The model under review builds one solid part; all positions refer to its coordinate system, in mm. Face numbers are marked on the shaded views. A direction names the side the tool comes from. Coordinates: 2 decimals unless noted, no trailing zeros. Write each loop counter-clockwise with the first axis right and the second up, starting at its lowest first coordinate (ties: lowest second). Pieces come first, ordered by that corner, then holes.
1) Add section C-C, the plane x = 25. State the section outline as (y, z) points.
2) Add section A-A, the plane y = -12.5. State the section outline as (x, z) points.
3) For P1, Ø10, axis at x = 25.5, z = 15, coming from the -Y side (3 decimals); P2, Ø1.2, axis at y = 1, z = 23.5, coming from the +X side; P3, Ø2, axis at y = 0.5, z = 25, coming from the -X side; P4, Ø8, axis at x = 18.5, y = -19, coming from the +Z side, all flat-tipped, find the tip position at first contact; note any pin that passes through.
4) Add section D-D, the plane z = 20. State the section outline as (x, y) points.
5) Mouldability with a two-part tool opening along Z and no side actions: class the marked faces 4, 5 and 6 as released by +Z, released by -Z, zero draft, split by the parting line, or undercut.
6) For line 1 (X direction, y = 12.5, z = 1.5); line 2 (Y direction, x = -25, z = 4); line 3 (Y direction, x = 0, z = 39.6), list the stretches that pass through material, from the lowest coordinate up.
7) Add section B-B, the plane z = 3. State the section outline as (x, y) points, then the cut area to 3 significant figures.
8) Machinability: for the marked faces 1, 2 and 3, which of the approach directions +Z, -Z, +X, -X, +Y, -Y give a long, thin tool a straight path to every point of the face, cutting with its end or side? Answer none if there is none.
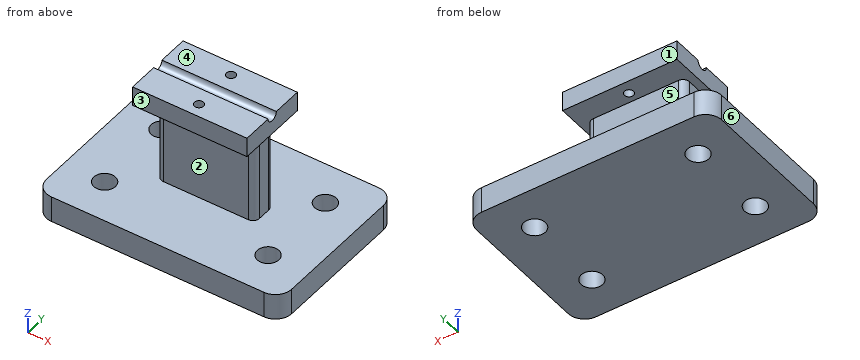
Autodesk Fusion 360 part; units mm, degrees
sketch "草图1" plane through (0, 0, 0) normal (0, 0, 1) x (1, 0, 0)
  line L0 (37.5, -25) -> (-37.5, -25)
  line L1 (-37.5, -25) -> (-37.5, 25)
  line L2 (-37.5, 25) -> (37.5, 25)
  line L3 (37.5, 25) -> (37.5, -25)
  line L4 (37.5, -25) -> (-37.5, 25) construction
  line L5 (-37.5, -25) -> (37.5, 25) construction
  dimension "d34" = 75
  dimension "d35" = 50
extrude "拉伸1" add sketch "草图1" along normal blind 8
fillet "圆角1" radius 5 4 edges at (37.5, -25, 4) (-37.5, -25, 4) (37.5, 25, 4) (-37.5, 25, 4)
sketch "草图2" plane through (0, 0, 8) normal (0, 0, 1) x (-1, 0, 0)
  arc A0 (32.5, -25) -> (37.5, -20) centre (32.5, -20) ccw
  line L0 (37.5, -20) -> (37.5, 20)
  arc A1 (37.5, 20) -> (32.5, 25) centre (32.5, 20) ccw
  line L1 (32.5, 25) -> (-32.5, 25)
  arc A2 (-32.5, 25) -> (-37.5, 20) centre (-32.5, 20) ccw
  line L2 (-37.5, 20) -> (-37.5, -20)
  arc A3 (-37.5, -20) -> (-32.5, -25) centre (-32.5, -20) ccw
  line L3 (-32.5, -25) -> (32.5, -25)
  point P0 (-25, -12.5)
  dimension "d40" = 12.5
  dimension "d41" = 12.5
hole "孔1" at (25, 12.5, 8) direction (0, 0, -1) diameter 6.6 depth 25 tip angle 180
pattern_linear "R-阵列1" count 2 spacing 50 along (-1, 0, 0) count 2 spacing 25 along (0, -1, 0) of "孔1"
sketch "草图3" plane through (0, 0, 8) normal (0, 0, 1) x (-1, 0, 0)
  circle A0 centre (25, 12.5) radius 3.3
  circle A1 centre (-25, 12.5) radius 3.3
  circle A2 centre (25, -12.5) radius 3.3
  circle A3 centre (-25, -12.5) radius 3.3
  arc A4 (32.5, -25) -> (37.5, -20) centre (32.5, -20) ccw
  line L0 (37.5, -20) -> (37.5, 20)
  arc A5 (37.5, 20) -> (32.5, 25) centre (32.5, 20) ccw
  line L1 (32.5, 25) -> (-32.5, 25)
  arc A6 (-32.5, 25) -> (-37.5, 20) centre (-32.5, 20) ccw
  line L2 (-37.5, 20) -> (-37.5, -20)
  arc A7 (-37.5, -20) -> (-32.5, -25) centre (-32.5, -20) ccw
  line L3 (-32.5, -25) -> (32.5, -25)
  line L4 (15, -4) -> (-15, -4)
  line L5 (-15, -4) -> (-15, 4)
  line L6 (-15, 4) -> (15, 4)
  line L7 (15, 4) -> (15, -4)
  line L8 (15, -4) -> (-15, 4) construction
  line L9 (-15, -4) -> (15, 4) construction
  dimension "d49" = 30
  dimension "d50" = 8
extrude "拉伸2" add sketch "草图3" along normal blind 27.5 contours L4 L5 L6 L7
sketch "草图4" plane through (0, 0, 35.5) normal (0, 0, 1) x (-1, 0, 0)
  line L0 (15, 4) -> (-15, 4)
  line L1 (-15, 4) -> (-15, -4)
  line L2 (-15, -4) -> (15, -4)
  line L3 (15, -4) -> (15, 4)
  line L4 (17.5, -11) -> (-17.5, -11)
  line L5 (-17.5, -11) -> (-17.5, 11)
  line L6 (-17.5, 11) -> (17.5, 11)
  line L7 (17.5, 11) -> (17.5, -11)
  line L8 (17.5, -11) -> (-17.5, 11) construction
  line L9 (-17.5, -11) -> (17.5, 11) construction
  dimension "d53" = 35
  dimension "d54" = 22
extrude "拉伸3" add sketch "草图4" along normal blind 6 contours L0 L1 L2 L3 | L4 L5 L6 L7
sketch "草图5" plane through (0, 0, 0) normal (1, 0, 0) x (0, 1, 0)
  line L0 (11, 41.5) -> (-11, 41.5)
  line L1 (11, 35.5) -> (11, 41.5)
  line L2 (-11, 35.5) -> (-11, 41.5)
  circle A0 centre (0, 41.5) radius 1.8
  dimension "d57" = 3.6
extrude "拉伸4" cut sketch "草图5" along normal blind 17.5 and the other way blind 17.5
sketch "草图6" plane through (0, 0, 41.5) normal (0, 0, 1) x (-1, 0, 0)
  line L0 (17.5, -1.8) -> (-17.5, -1.8)
  line L1 (-17.5, -1.8) -> (-17.5, -11)
  line L2 (-17.5, -11) -> (17.5, -11)
  line L3 (17.5, -11) -> (17.5, -1.8)
  point P0 (0, 7)
  point P1 (0, -7)
hole "孔2" at (0, -7, 41.5) at (0, 7, 41.5) direction (0, 0, -1) diameter 2.8 depth 10 tip angle 118
fillet "圆角2" radius 2 4 edges at (15, 4, 21.75) (-15, 4, 21.75) (15, -4, 21.75) (-15, -4, 21.75)
component "Fixed_Catheter_Clamp_Base" placed x (1, 0, 0) y (0, 1, 0) z (0, 0, 1) at (0, 0, 0)
equation "Rail_Support_Height = 8 mm"
equation "MGN12H_Combined_Height = 13 mm"
equation "Pulley_Base_Thickness = 6 mm"
equation "Wheel_Base_Clearance = 1.5 mm"
equation "Pulley_Groove_Center_Height = 8 mm"
equation "Clamp_Base_Length = 75 mm"
equation "Clamp_Base_Width = 50 mm"
equation "Clamp_Base_Thickness = 8 mm"
equation "Clamp_Base_Corner_Radius = 5 mm"
equation "Table_Hole_Pitch_X = 50 mm"
equation "Table_Hole_Pitch_Y = 25 mm"
equation "M6_Clearance_Diameter = 6.6 mm"
equation "Column_Length = 30 mm"
equation "Column_Width = 20 mm"
equation "Lower_Jaw_Length = 35 mm"
equation "Lower_Jaw_Width = 22 mm"
equation "Lower_Jaw_Height = 6 mm"
equation "Upper_Jaw_Length = 35 mm"
equation "Upper_Jaw_Width = 22 mm"
equation "Upper_Jaw_Height = 5 mm"
equation "Catheter_Diameter = 2.4 mm"
equation "Ecoflex_Pad_Nominal_Thickness = 0.5 mm"
equation "Catheter_Assembly_Clearance = 0.2 mm"
equation "Clamp_M3_Offset_Y = 7 mm"
equation "M3_Cap_Clearance_Diameter = 3.4 mm"
equation "M3_Lower_Pilot_Diameter = 2.8 mm"
equation "M3_Lower_Pilot_Depth = 5 mm"
equation "Column_Base_Fillet = 4 mm"
equation "Jaw_Column_Fillet = 2 mm"
equation "Edge_Fillet = 1 mm"
equation "d34 = Clamp_Base_Length"
equation "d35 = Clamp_Base_Width"
equation "d36 = Clamp_Base_Thickness"
equation "d39 = Clamp_Base_Corner_Radius"
equation "d43 = M6_Clearance_Diameter"
equation "d49 = Column_Length"
equation "d50 = Column_Width / 2 - 2 mm"
equation "d51 = Column_Height + 5 mm"
equation "d53 = Lower_Jaw_Length"
equation "d54 = Lower_Jaw_Width"
equation "d55 = Lower_Jaw_Height"
equation "d57 = Clamp_Groove_Diameter"
equation "d62 = M3_Lower_Pilot_Depth + 5 mm"
equation "d63 = M3_Lower_Pilot_Diameter"
equation "d66 = Jaw_Column_Fillet"
Geometry results:
1. outline: (-25, 0) - (-15.8, 0) - (-15.8, 8) - (-25, 8) - close; (-9.2, 0) - (9.2, 0) - (9.2, 8) - (-9.2, 8) - close; (15.8, 0) - (25, 0) - (25, 8) - (15.8, 8) - close
2. outline: (-37.5, 0) - (-28.3, 0) - (-28.3, 8) - (-37.5, 8) - close; (-21.7, 0) - (21.7, 0) - (21.7, 8) - (-21.7, 8) - close; (28.3, 0) - (37.5, 0) - (37.5, 8) - (28.3, 8) - close
3. P1: passes through
3. P2: stops at x = 15
3. P3: stops at x = -15
3. P4: stops at z = 8
4. outline: (-15, -2) arc R2 ccw to (-13, -4) - (13, -4) arc R2 ccw to (15, -2) - (15, 2) arc R2 ccw to (13, 4) - (-13, 4) arc R2 ccw to (-15, 2) - close
5. face 4: released by +Z
5. face 5: undercut
5. face 6: zero draft
6. line 1: x = -37.5 to -28.3, -21.7 to 21.7, 28.3 to 37.5
6. line 2: y = -25 to -15.8, -9.2 to 9.2, 15.8 to 25
6. line 3: y = -11 to -8.4, -5.6 to 5.6, 8.4 to 11
7. outline: (-37.5, -20) arc R5 ccw to (-32.5, -25) - (32.5, -25) arc R5 ccw to (37.5, -20) - (37.5, 20) arc R5 ccw to (32.5, 25) - (-32.5, 25) arc R5 ccw to (-37.5, 20) - close; hole circle Ø6.6 at (-25, -12.5); hole circle Ø6.6 at (-25, 12.5); hole circle Ø6.6 at (25, -12.5); hole circle Ø6.6 at (25, 12.5)
7. area: 3,590 mm2
8. face 1: +Z, +X, -X, +Y
8. face 2: +X, -X, -Y
8. face 3: +Z, +X, -X, -Y
